Design review of the part built by this model. Coordinates are the model's own, in mm. Round coordinates to 2 decimals unless told otherwise and drop trailing zeros. Loops run counter-clockwise (first coordinate to the right, second up) from the corner with the lowest first, then second, coordinate; pieces in that order, holes last. Notation, with made-up numbers: (-23.5, 37) - (15.5, 37) arc R13 ccw to (15.5, 48) - close; hole circle Ø10 at (51, 72). An arc over 180 degrees is marked (long way). Return JSON: item names as keys, results as strings. Group by question number.
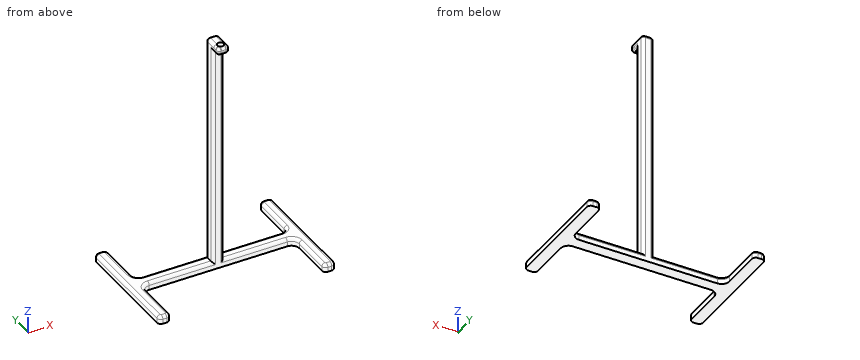
from build123d import *

# Parameters (mm, degrees)
SKETCH_W     = 100
SKETCH_H     = 7.5
PAD_DEPTH    = 5
FILLET_R     = 5
SKETCH001_W  = 7.5
SKETCH001_H  = 7.5
PAD001_DEPTH = 150
SKETCH002_W  = 7.5
SKETCH002_H  = 5
PAD002_DEPTH = 10
SKETCH003_R  = 2.1
POCKET_DEPTH = 5
FILLET001_R  = 2


with BuildPart() as part:
    # Sketch → Pad (new body)
    with BuildSketch(Plane.XY):
        Rectangle(SKETCH_W, SKETCH_H)
        with BuildLine():
            Line((50, 35), (50, -35))
            ThreePointArc((50, -35), (50.732233, -36.767767), (52.5, -37.5))
            Line((52.5, -37.5), (55, -37.5))
            ThreePointArc((55, -37.5), (56.767767, -36.767767), (57.5, -35))
            Line((57.5, -35), (57.5, 35))
            ThreePointArc((57.5, 35), (56.767767, 36.767767), (55, 37.5))
            Line((55, 37.5), (52.5, 37.5))
            ThreePointArc((52.5, 37.5), (50.732233, 36.767767), (50, 35))
        make_face()
        with BuildLine():
            Line((-52.5, 37.5), (-55, 37.5))
            ThreePointArc((-55, 37.5), (-56.767767, 36.767767), (-57.5, 35))
            Line((-57.5, 35), (-57.5, -35))
            ThreePointArc((-57.5, -35), (-56.767767, -36.767767), (-55, -37.5))
            Line((-55, -37.5), (-52.5, -37.5))
            ThreePointArc((-52.5, -37.5), (-50.732233, -36.767767), (-50, -35))
            Line((-50, -35), (-50, 35))
            ThreePointArc((-50, 35), (-50.732233, 36.767767), (-52.5, 37.5))
        make_face()
    extrude(amount=PAD_DEPTH)

    # Fillet
    fillet_edges = [part.edges().sort_by_distance(p)[0] for p in [
        (-50, -3.75, 2.5),
        (50, -3.75, 2.5),
        (-50, 3.75, 2.5),
        (50, 3.75, 2.5),
    ]]
    fillet(fillet_edges, radius=FILLET_R)

    # Sketch001 (on Face5 of Fillet) → Pad001 (join)
    with BuildSketch(Plane.XY.offset(5)):
        Rectangle(SKETCH001_W, SKETCH001_H)
    extrude(amount=PAD001_DEPTH)

    # Sketch002 → Pad002 (join)
    with BuildSketch(Plane.XZ):
        with Locations((0, 152.5)):
            Rectangle(SKETCH002_W, SKETCH002_H)
    extrude(amount=PAD002_DEPTH)

    # Sketch003 (on Face32 of Pad002) → Pocket (cut)
    with BuildSketch(Plane.XY.offset(155)):
        with Locations((0, -6.4)):
            Circle(SKETCH003_R)
    extrude(amount=-POCKET_DEPTH, mode=Mode.SUBTRACT)

    # Fillet001
    fillet001_edges = [part.edges().sort_by_distance(p)[0] for p in [
        (-50, -21.875, 5),
        (-3.75, -3.75, 77.5),
        (24.375, -3.75, 5),
        (3.75, -3.75, 77.5),
        (-3.75, 3.75, 80),
        (3.75, 3.75, 80),
        (0, -10, 155),
        (3.75, -3.125, 155),
        (-3.75, -3.125, 155),
        (0, 3.75, 155),
        (3.75, -6.875, 150),
        (3.75, -10, 152.5),
        (0, -10, 150),
        (-3.75, -10, 152.5),
        (-3.75, -6.875, 150),
    ]]
    fillet(fillet001_edges, radius=FILLET001_R)


solid = part.part
Q1. Add section B-B, the plane z = 99. State the section outline as (x, y) points, plus the area to 3 significant figures.
Q2. Insertion check: pin 1 Ø6 at (y, z) = (0, 28) entering from +X; pin 2 Ø3 at (x, y) = (26.5, -2) entering from +Z; pin 3 Ø3 at (y, z) = (-5, 99.5) entering from -X; pin 4 Ø1.6 at (x, y) = (0.5, -4.5) entering from -Z. Each pin has a flat end and moves straight along its axis. Give the tip position at first contact, or say it passes through.
Q3. For line 1 (X direction, y = -6.4, z = 153.05); line 2 (Y direction, x = 0, z = 151.55), list the stretches that pass through material, from the lowest coordinate up.
Q4. Add section A-A, the plane y = 16.5. State the section outline as (x, z) points, plus the area to 3 significant figures.
Q5. Add section C-C, the plane x = -38.5. State the section outline as (y, z) points, plus the area to 3 significant figures.
Evaluation:
{
 "1": {"outline": "(-3.75, -1.75) arc R2 ccw to (-1.75, -3.75) - (1.75, -3.75) arc R2 ccw to (3.75, -1.75) - (3.75, 1.75) arc R2 ccw to (1.75, 3.75) - (-1.75, 3.75) arc R2 ccw to (-3.75, 1.75) - close", "area": "52.8 mm²"},
 "2": {"pin 1": "x = 3.75", "pin 2": "z = 5", "pin 3": "x = -2.72", "pin 4": "z = 0"},
 "3": {"line 1": "-3.75 to -2.1, 2.1 to 3.75", "line 2": "-9.96 to -8.5, -4.3 to 3.75"},
 "4": {"outline": "(-57.5, 0) - (-50, 0) - (-50, 3) arc R2 ccw to (-52, 5) - (-55.5, 5) arc R2 ccw to (-57.5, 3) - close; (50, 0) - (57.5, 0) - (57.5, 3) arc R2 ccw to (55.5, 5) - (52, 5) arc R2 ccw to (50, 3) - close", "area": "71.6 mm²"},
 "5": {"outline": "(-3.75, 0) - (3.75, 0) - (3.75, 3) arc R2 ccw to (1.75, 5) - (-1.75, 5) arc R2 ccw to (-3.75, 3) - close", "area": "35.8 mm²"}
}
